Autodesk Inventor part; units mm, degrees
ref_plane "YZ Plane" through (0, 0, 0) normal (1, 0, 0) x (0, 1, 0)
ref_plane "XZ Plane" through (0, 0, 0) normal (0, 1, 0) x (-1, 0, 0)
ref_plane "XY Plane" through (0, 0, 0) normal (0, 0, 1) x (1, 0, 0)
sketch "Sketch1" plane through (0, 0, 0) normal (0, 0, 1) x (1, 0, 0)
  circle A0 centre (0, 0) radius 2.5
  dimension "d0" = 5
extrude "Extrusion1" add sketch "Sketch1" along normal blind 25
sketch "Sketch2" plane through (0, 0, 25) normal (0, 0, 1) x (1, 0, 0)
  circle A0 centre (0, 0) radius 2.5
  line L0 (2.5, 0) -> (-2, 0)
  line L1 (-2, 0) -> (-2, 4)
  line L2 (-2, 0) -> (-2, -4)
  line L3 (-2, -4) -> (-6, -4)
  line L4 (-6, -4) -> (-6, 4)
  line L5 (-6, 4) -> (-2, 4)
  point P0 (-2, -1.5)
  point P1 (-2, 1.5)
  dimension "d3" = 4.5
  dimension "d6" = 4
  dimension "d7" = 4
  dimension "d8" = 4
extrude "Extrusion2" cut sketch "Sketch2" against normal blind 15 contours A0 L2 L3 L4 L5 L1
extrude "Extrusion3" cut sketch "Sketch2" against normal blind 15 contours L1 L2 A0
properties part number "AXE"
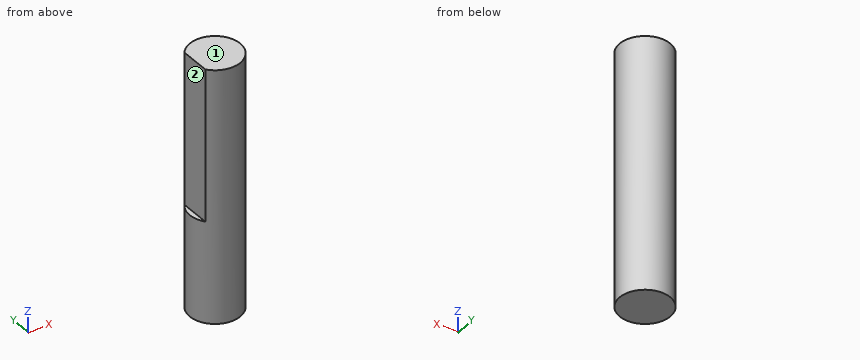
For this review, take the finished solid that the model builds, in its own axes (mm). Face numbers are marked on the shaded views. A direction names the side the tool comes from. Coordinates: 2 decimals unless noted, no trailing zeros. Order: outer loops, then holes, each group sorted by start corner. A loop starts at its lowest first (then second) coordinate and runs counter-clockwise, first axis right, second up. Notation, with made-up numbers: (8.25, 78) - (56.25, 78) arc R19 cw to (56.25, 86) - close; hole circle Ø6 at (-40, 12.25). An arc over 180 degrees is marked (long way). Answer as a JSON object with one key per item and string values. Group by question number.
1. We need section A-A on y = -1.25. State the section outline as (x, z) points, then the cut area to 3 significant figures.
2. We need section B-B on z = 5. State the section outline as (x, y) points.
3. We need section D-D on y = 0. State the section outline as (x, z) points.
4. For the marked faces 1 and 2, list the 3-axis set-ups (+Z, -Z, +X, -X, +Y, -Y) from which the entire face can be reached by the end or side of a thin tool; tool diameter is ignored.
5. Clearance check with a flat-ended pin moving along its axis: P1, Ø1.5, axis at y = 0.5, z = 17, coming from the -X side. State where the tip first meets the part, or that it passes through.
6. For probe 1 along Z at (x, y) = (-2.1, 1.2); probe 2 along Y at (x, z) = (-0.1, 6.25); probe 3 along X at (y, z) = (-2, 19.25), list the stretches that pass through material, from the lowest coordinate up.
7. We need section C-C on x = -1.4. State the section outline as (y, z) points.
Final values:
{
 "1": {"outline": "(-2.17, 0) - (2.17, 0) - (2.17, 25) - (-2, 25) - (-2, 10) - (-2.17, 10) - close", "area": "106 mm²"},
 "2": {"outline": "circle Ø5 at (0, 0)"},
 "3": {"outline": "(-2.5, 0) - (2.5, 0) - (2.5, 25) - (-2, 25) - (-2, 10) - (-2.5, 10) - close"},
 "4": {"face 1": "+Z, +X, -X, +Y, -Y", "face 2": "+Z, -X, +Y, -Y"},
 "5": {"P1": "x = -2"},
 "6": {"probe 1": "0 to 10", "probe 2": "-2.5 to 2.5", "probe 3": "-1.5 to 1.5"},
 "7": {"outline": "(-2.07, 0) - (2.07, 0) - (2.07, 25) - (-2.07, 25) - close"}
}
